Autodesk Inventor part; units mm, degrees
ref_plane "YZ Plane" through (0, 0, 0) normal (1, 0, 0) x (0, 1, 0)
ref_plane "XZ Plane" through (0, 0, 0) normal (0, 1, 0) x (-1, 0, 0)
ref_plane "XY Plane" through (0, 0, 0) normal (0, 0, 1) x (1, 0, 0)
sketch "Sketch1" plane through (0, 0, 0) normal (0, 0, 1) x (1, 0, 0)
  circle A0 centre (0, 0) radius 51
  dimension "d0" = 102
extrude "Extrusion1" add sketch "Sketch1" along normal blind 5
sketch "Sketch2" plane through (0, 0, 0) normal (0, 0, -1) x (-1, 0, 0)
  line L0 (0, 5.7735) -> (5, 2.8868)
  line L1 (5, 2.8868) -> (5, -2.8868)
  line L2 (5, -2.8868) -> (0, -5.7735)
  line L3 (0, -5.7735) -> (-5, -2.8868)
  line L4 (-5, -2.8868) -> (-5, 2.8868)
  line L5 (-5, 2.8868) -> (0, 5.7735)
  point P0 (0, 0)
  point P1 (0, 0)
  dimension "d3" = 10
extrude "Extrusion2" cut sketch "Sketch2" against normal blind 5
sketch "Sketch3" plane through (0, 0, 0) normal (0, 0, -1) x (-1, 0, 0)
  circle A0 centre (0, 0) radius 15 construction
  point P0 (0, 15)
  point P1 (15, 0)
  point P2 (0, -15)
  point P3 (-15, 0)
  dimension "d6" = 30
hole "Hole1" at (0, 15, 0) at (-15, 0, 0) at (0, -15, 0) at (15, 0, 0) direction (0, 0, 1) diameter 3.4 depth 8 tip angle 118
sketch "Sketch4" plane through (0, 0, 0) normal (0, 0, -1) x (-1, 0, 0)
  line L0 (-1.6, 51) -> (1.6, 51)
  line L1 (1.6, 51) -> (1.6, 46)
  line L2 (1.6, 46) -> (-2.75, 46)
  line L3 (-2.75, 46) -> (-2.75, 43.6)
  line L4 (-2.75, 43.6) -> (2.75, 43.6)
  line L5 (2.75, 43.6) -> (2.75, 46)
  line L6 (2.75, 46) -> (-1.6, 46)
  line L7 (-1.6, 46) -> (-1.6, 51)
  line L8 (-51, -1.6) -> (-51, 1.6)
  line L9 (-51, 1.6) -> (-46, 1.6)
  line L10 (-46, 1.6) -> (-46, -2.75)
  line L11 (-46, -2.75) -> (-43.6, -2.75)
  line L12 (-43.6, -2.75) -> (-43.6, 2.75)
  line L13 (-43.6, 2.75) -> (-46, 2.75)
  line L14 (-46, 2.75) -> (-46, -1.6)
  line L15 (-46, -1.6) -> (-51, -1.6)
  line L16 (1.6, -51) -> (-1.6, -51)
  line L17 (-1.6, -51) -> (-1.6, -46)
  line L18 (-1.6, -46) -> (2.75, -46)
  line L19 (2.75, -46) -> (2.75, -43.6)
  line L20 (2.75, -43.6) -> (-2.75, -43.6)
  line L21 (-2.75, -43.6) -> (-2.75, -46)
  line L22 (-2.75, -46) -> (1.6, -46)
  line L23 (1.6, -46) -> (1.6, -51)
  line L24 (51, 1.6) -> (51, -1.6)
  line L25 (51, -1.6) -> (46, -1.6)
  line L26 (46, -1.6) -> (46, 2.75)
  line L27 (46, 2.75) -> (43.6, 2.75)
  line L28 (43.6, 2.75) -> (43.6, -2.75)
  line L29 (43.6, -2.75) -> (46, -2.75)
  line L30 (46, -2.75) -> (46, 1.6)
  line L31 (46, 1.6) -> (51, 1.6)
  point P0 (0, 0)
  point P1 (0, 43.6)
  point P2 (0, 51)
  point P3 (-51, 0)
  point P4 (-43.6, 0)
  point P5 (0, -51)
  point P6 (0, -43.6)
  point P7 (51, 0)
  point P8 (43.6, 0)
  dimension "d14" = 5
  dimension "d15" = 2.4
  dimension "d16" = 5.5
  dimension "d17" = 3.2
  dimension "d18" = 51
  dimension "d21" = 360
extrude "Extrusion3" cut sketch "Sketch4" against normal through all
properties part number "PlexiHalter1" material "Polycarbonate, Clear"
For this review, take the finished solid that the model builds, in its own axes (mm). A direction names the side the tool comes from. Give positions to 0.01 mm unless a question says otherwise; leave off trailing zeros. Order: outer loops, then holes, each group sorted by start corner. A loop starts at its lowest first (then second) coordinate and runs counter-clockwise, first axis right, second up. Notation, with made-up numbers: (33, -13.5) - (73, -13.5) arc R34 cw to (73, 21.5) - close; hole circle Ø7 at (-14.5, -3). An arc over 180 degrees is marked (long way). Answer as a JSON object with one key per item and string values. Group by question number.
Item 1: Draft analysis for pull direction X (two halves, no side actions). For faces 4 (the flat face through (11, 1, 0)), 5 (the cylindrical face through (36.44, -35.68, 2.46)), 6 (the flat face through (-1.6, -48, 2)), state which applies: pulls with the +X half, pulls with the -X half, needs draft (parallel to the pull), parting line crosses it, or undercut.
Item 2: Clearance check with flat-ended pins moving along their axes: pin 1 Ø1.9 at (x, z) = (-44.5, 1.5) entering from +Y; pin 2 Ø1.5 at (x, z) = (-47.5, 3) entering from +Y; pin 3 Ø1.5 at (x, z) = (20, 2) entering from -Y; pin 4 Ø5 at (x, y) = (-38.5, 37.5) entering from -Z. State where each tip first meets the part, or that it passes through.
Item 3: Machinability: for faces 1 (the flat face through (-1.6, 49, 2)), 2 (the flat face through (5, 0, 2)), 3 (the flat face through (-49, -1.6, 2)), which of the approach directions +Z, -Z, +X, -X, +Y, -Y give a long, thin tool a straight path to every point of the face, cutting with its end or side? Answer none if there is none.
Item 4: Wall thickness on line 1 along X through (y, z) = (0, 2.35); line 2 along Y through (x, z) = (0, 3); line 3 along Y through (x, z) = (-22, 2.4): over which ranges is each line inside the solid? List them lowest first.
Item 5: Take a section at A-A on y = 0. Give the boundary of the cut face in (x, z).
Item 6: Take a section at B-B on x = 15. Give the boundary of the cut face in (y, z), and give its area (3 significant figures).
Item 7: Take a section at C-C on z = 3.1. Give the number of separate pieces and of enclosed holes in the cut face, and give its area (3 significant figures).
Reported:
{
 "1": {"face 4": "needs draft", "face 5": "pulls with the +X half", "face 6": "undercut"},
 "2": {"pin 1": "y = 26.54", "pin 2": "y = 20.38", "pin 3": "y = -47.23", "pin 4": "through"},
 "3": {"face 1": "+Z, -Z, +Y", "face 2": "+Z, -Z", "face 3": "+Z, -Z, -X"},
 "4": {"line 1": "-43.6 to -16.7, -13.3 to -5, 5 to 13.3, 16.7 to 43.6", "line 2": "-43.6 to -16.7, -13.3 to -5.77, 5.77 to 13.3, 16.7 to 43.6", "line 3": "-46.01 to 46.01"},
 "5": {"outline": "(-43.6, 0) - (-16.7, 0) - (-16.7, 5) - (-43.6, 5) - close; (-13.3, 0) - (-5, 0) - (-5, 5) - (-13.3, 5) - close; (5, 0) - (13.3, 0) - (13.3, 5) - (5, 5) - close; (16.7, 0) - (43.6, 0) - (43.6, 5) - (16.7, 5) - close"},
 "6": {"outline": "(-48.74, 0) - (-1.7, 0) - (-1.7, 5) - (-48.74, 5) - close; (1.7, 0) - (48.74, 0) - (48.74, 5) - (1.7, 5) - close", "area": "470 mm^2"},
 "7": {"separate pieces": "1", "enclosed holes": "5", "area": "7,930 mm^2"}
}
